Geometry check sheet. Reference: the model listing, model coordinates, mm. A direction names the side the tool comes from. Coordinates: 2 decimals unless noted, no trailing zeros. Write each loop counter-clockwise with the first axis right and the second up, starting at its lowest first coordinate (ties: lowest second). Pieces come first, ordered by that corner, then holes. Notation, with made-up numbers: M 19,-34 L 31,-34 A29 cw 31,-3 Z; hole C 45.25,-33.75 d10. An arc over 180 degrees is marked long. Put each result on its own line as item: value. Start each with the question number.
1) Set-up check for faces 1 (the flat face through (20, -27, 2)), 2 (the flat face through (20, 27, 2)), 3 (the flat face through (-20, -27, 2)), 4 (the flat face through (-30, 25, 2)): record each of +Z, -Z, +X, -X, +Y, -Y from which the full face is reachable in a straight line by a thin tool's end or side.
2) Cross-section at C-C on x = 13.5. Record the cut outline in (y, z).
3) Scan lines: line 1 along Y through (x, z) = (-15, 1.4); line 2 along Y through (x, z) = (12, 1.55); line 3 along X through (y, z) = (14.5, 0.35). Record each from-to range of solid material in increasing order.
4) Cross-section at B-B on z = 1.5. Record the cut outline in (x, y).
5) Gauge pin test, flat ends, axial feed: pin 1 (10.5 mm diameter, centred on x = -15, y = 15.5, fed in from -Z); pin 2 (2 mm diameter, centred on x = 27, z = 1.5, fed in from -Y); pin 3 (2 mm diameter, centred on x = -25, z = 1.5, fed in from +Y); pin 4 (1.2 mm diameter, centred on y = -27.5, z = 1.5, fed in from -X). Record the tip position at first contact, or that the pin passes through.
6) Cross-section at A-A on y = 15.5. Record the cut outline in (x, z), plus the area to 3 significant figures.
7) Mould release check, pull along Y, two halves, no side actions. Record for faces 5 (the flat face through (0, 29, 2)), 6 (the cylindrical face through (-12.05, 12.8, 1.97)), 7 (the flat face through (30, -25, 2)), 8 (the flat face through (40, 0, 2)): released by +Y, released by -Y, zero draft, split by the parting line, or undercut.
from build123d import *

# Parameters (mm, degrees)
SKETCH1_R           = 4
BOSS_EXTRUDE1_DEPTH = 4


with BuildPart() as part:
    # Sketch1 → Boss-Extrude1 (new body)
    with BuildSketch(Plane.XY):
        Polygon((-20, 29), (20, 29), (20, 25), (40, 25), (40, -25), (20, -25), (20, -29), (-20, -29), (-20, -25), (-40, -25), (-40, 25), (-20, 25), align=None)
        with Locations((15, 15.5)):
            Circle(SKETCH1_R, mode=Mode.SUBTRACT)
        with Locations(Location((-15, 15.5, 0), (0, 0, 180))):
            Circle(SKETCH1_R, mode=Mode.SUBTRACT)
        with Locations((-15, -15.5)):
            Circle(SKETCH1_R, mode=Mode.SUBTRACT)
        with Locations(Location((15, -15.5, 0), (0, 0, 180))):
            Circle(SKETCH1_R, mode=Mode.SUBTRACT)
    extrude(amount=BOSS_EXTRUDE1_DEPTH)


solid = part.part
Answer key:
1. face 1: +Z, -Z, +X, -Y
1. face 2: +Z, -Z, +X, +Y
1. face 3: +Z, -Z, -X, -Y
1. face 4: +Z, -Z, -X, +Y
2. outline: M -29,0 L -19.21,0 L -19.21,4 L -29,4 Z; M -11.79,0 L 11.79,0 L 11.79,4 L -11.79,4 Z; M 19.21,0 L 29,0 L 29,4 L 19.21,4 Z
3. line 1: y = -29 to -19.5, -11.5 to 11.5, 19.5 to 29
3. line 2: y = -29 to -18.15, -12.85 to 12.85, 18.15 to 29
3. line 3: x = -40 to -18.87, -11.13 to 11.13, 18.87 to 40
4. outline: M -40,-25 L -20,-25 L -20,-29 L 20,-29 L 20,-25 L 40,-25 L 40,25 L 20,25 L 20,29 L -20,29 L -20,25 L -40,25 Z; hole C -15,-15.5 d8; hole C -15,15.5 d8; hole C 15,-15.5 d8; hole C 15,15.5 d8
5. pin 1: stops at z = 0
5. pin 2: stops at y = -25
5. pin 3: stops at y = 25
5. pin 4: stops at x = -20
6. outline: M -40,0 L -19,0 L -19,4 L -40,4 Z; M -11,0 L 11,0 L 11,4 L -11,4 Z; M 19,0 L 40,0 L 40,4 L 19,4 Z
6. area: 256 mm²
7. face 5: released by +Y
7. face 6: undercut
7. face 7: released by -Y
7. face 8: zero draft
